Design review of the part built by this model. Coordinates are the model's own, in mm. Face numbers are marked on the shaded views. A direction names the side the tool comes from. Round coordinates to 2 decimals unless told otherwise and drop trailing zeros. Loops run counter-clockwise (first coordinate to the right, second up) from the corner with the lowest first, then second, coordinate; pieces in that order, holes last. Notation, with made-up numbers: (75.5, -21) -> (91.5, -21) arc R35 cw to (91.5, 16) -> close; hole circle Ø2 at (-11.75, -9.75). An arc over 180 degrees is marked (long way). Answer as CSV lines item,"result". Start each with the question number.
(1) For P1, Ø3, axis at x = 99.5, y = 21, coming from the +Z side; P2, Ø1, axis at y = 12.5, z = -22, coming from the -X side; P3, Ø2, axis at x = 173.9, z = -21.5, coming from the +Y side; P4, Ø6.5, axis at x = 173, z = -20, coming from the +Y side, all flat-tipped, find the tip position at first contact; note any pin that passes through.
(2) Machinability: for the marked faces 1 and 2, which of the approach directions +Z, -Z, +X, -X, +Y, -Y give a long, thin tool a straight path to every point of the face, cutting with its end or side? Answer none if there is none.
(3) Take a section at C-C, the plane x = 83. Write out the cut boundary in (y, z).
(4) To check wall thickness, follow line 1 (Y direction, x = 153.5, z = -15.5); line 2 (Z direction, x = 141, y = 21.75); line 3 (X direction, y = 21.75, z = -8.75) (3 decimals). State the ranges of each line that lie inside material, in increasing order. Write a range as from..to.
(5) Take a section at A-A, the plane z = -21.5. Write out the cut boundary in (x, y), and give its area (3 significant figures).
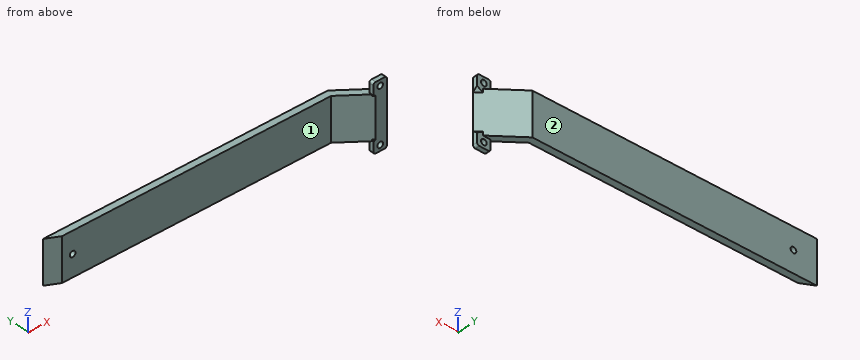
Autodesk Inventor part; units mm, degrees
ref_plane "YZ Plane" through (0, 0, 0) normal (1, 0, 0) x (0, 1, 0)
ref_plane "XZ Plane" through (0, 0, 0) normal (0, 1, 0) x (-1, 0, 0)
ref_plane "XY Plane" through (0, 0, 0) normal (0, 0, 1) x (1, 0, 0)
sketch "Эскиз1" plane through (0, 0, 0) normal (0, 0, 1) x (1, 0, 0)
  line L0 (176.9, 11.5) -> (160.5, 11.5)
  line L1 (19.5, 13.5) -> (19.5, 3.5)
  line L2 (19.5, 3.5) -> (127.2, 3.5)
  line L3 (127.2, 3.5) -> (127.2, -1.5)
  line L4 (127.2, -1.5) -> (2.5, -1.5)
  line L5 (2.5, -1.5) -> (2.5, 18.5)
  line L6 (2.5, 18.5) -> (36.5, 18.5)
  line L7 (36.5, 18.5) -> (36.5, 13.5)
  line L8 (36.5, 13.5) -> (19.5, 13.5)
  line L9 (131.9067, -6.5) -> (131.9067, 11.5)
  line L10 (131.9067, 11.5) -> (59.18, 11.5)
  line L11 (59.18, 11.5) -> (51.5, 15.5635)
  line L12 (36.5, 23.5) -> (-2.5, 23.5)
  line L13 (-2.5, 23.5) -> (-2.5, 12.5)
  line L14 (-2.5, 12.5) -> (0.5, 12.5)
  line L15 (0.5, 12.5) -> (0.5, 9.5)
  line L16 (0.5, 9.5) -> (-2.5, 9.5)
  line L17 (-2.5, 9.5) -> (-2.5, -3.5)
  line L18 (5.5, -6.5) -> (131.9067, -6.5)
  circle A0 centre (129.7, 9) radius 1.25
  line L19 (36.5, 23.5) -> (161.5, 23.5)
  line L20 (161.5, 23.5) -> (176.9, 11.5)
  line L21 (176.9, 11.5) -> (171.9, 11.5)
  line L22 (171.9, 11.5) -> (160.35, 20.5)
  line L23 (36.5, 23.5) -> (36.5, 20.5)
  line L24 (36.5, 20.5) -> (160.35, 20.5)
  line L25 (42.17, 20.5) -> (36.5, 23.5)
  line L26 (51.5, 20.5) -> (51.5, 15.5635)
  line L27 (42.17, 20.5) -> (51.5, 20.5)
  line L28 (5.5, -6.5) -> (5.5, -3.5)
  line L29 (-2.5, -3.5) -> (5.5, -3.5)
  point P0 (0, 0)
  point P1 (42.17, 20.5)
  dimension "d0" = 125
  dimension "d1" = 5
  dimension "d2" = 3
extrude "Выдавливание1" add sketch "Эскиз1" against normal blind 19 contours L0 L22 L24 L25 L19 L20 | L25 L24 L23
sketch "Эскиз2" plane through (36.5, 23.5, 0) normal (0, 1, 0) x (1, 0, 0)
  line L0 (125, 0) -> (0, 0)
  line L1 (0, 19) -> (125, 19)
  line L2 (0, 0) -> (10.335, 0) construction
  line L3 (10.335, 0) -> (10.335, 19) construction
  line L4 (10.335, 19) -> (0, 19) construction
  line L5 (0, 19) -> (0, 0) construction
  circle A0 centre (10.335, 9.5) radius 1.25
  point P0 (-36.5, 0)
  dimension "d5" = 10.335
  dimension "d6" = 2.5
extrude "Выдавливание2" cut sketch "Эскиз2" against normal blind 3
sketch "Эскиз3" plane through (171.9, 11.5, 0) normal (0, -1, 0) x (1, 0, 0)
  line L0 (5, 0) -> (-10.4, 0)
  line L1 (5, 0) -> (-1, 0)
  line L2 (-1, 0) -> (-1, 5)
  line L3 (-1, 5) -> (5, 5)
  line L4 (5, 5) -> (5, 0)
  line L5 (-1, 2.5) -> (5, 2.5) construction
  line L6 (2, 5) -> (2, 0) construction
  circle A0 centre (2, 2.5) radius 1.25
  line L7 (5, 0) -> (5, -19) construction
  line L8 (5, 0) -> (5, -19) construction
  line L9 (5, 0) -> (5, -19) construction
  line L10 (5, -9.5) -> (-10.4, -9.5) construction
  line L11 (-10.4, 0) -> (-10.4, -19) construction
  line L12 (5, -19) -> (-1, -19)
  line L13 (-1, -19) -> (-1, -24)
  line L14 (-1, -24) -> (5, -24)
  line L15 (5, -24) -> (5, -19)
  line L16 (-1, -21.5) -> (5, -21.5) construction
  line L17 (2, -24) -> (2, -19) construction
  circle A1 centre (2, -21.5) radius 1.25
  point P0 (-171.9, 0)
  point P1 (-1, 0)
  dimension "d9" = 6
  dimension "d10" = 5
  dimension "d11" = 2.5
extrude "Выдавливание3" add sketch "Эскиз3" against normal blind 2
chamfer "Фаска1" distance 1.5775 angle 45 2 edges at (175.6167, 12.5, -19) (175.6167, 12.5, 0)
fillet "Сопряжение1" radius 1 4 edges at (170.9, 12.5, 5) (176.9, 12.5, 5) (176.9, 12.5, -24) (170.9, 12.5, -24)
chamfer "Фаска2" distance 5.7 distance2 3 1 edges at (36.5, 20.5, -9.5) measured on face at (122.9283, 20.5, -9.5)
chamfer "Фаска3" distance 0.614 angle 45 2 edges at (171.4, 11.8896, 0) (171.4, 11.8896, -19)
properties part number "handle"
The answers:
1,P1,"z = 0"
1,P2,"x = 170.9"
1,P3,"through"
1,P4,"y = 16.95"
2,face 1,"+Z, -Z, -X, -Y"
2,face 2,"+Z, -Z, +X, -X, +Y"
3,outline,"(20.5, -19) -> (23.5, -19) -> (23.5, 0) -> (20.5, 0) -> close"
4,line 1,"20.5..23.5"
4,line 2,"-19..0"
4,line 3,"39.824..45.835, 47.835..163.746"
5,outline,"(170.9, 11.5) -> (172.65, 11.5) -> (172.65, 13.5) -> (170.9, 13.5) -> close; (175.15, 11.5) -> (176.9, 11.5) -> (176.9, 13.5) -> (175.15, 13.5) -> close"
5,area,"7.00 mm²"
